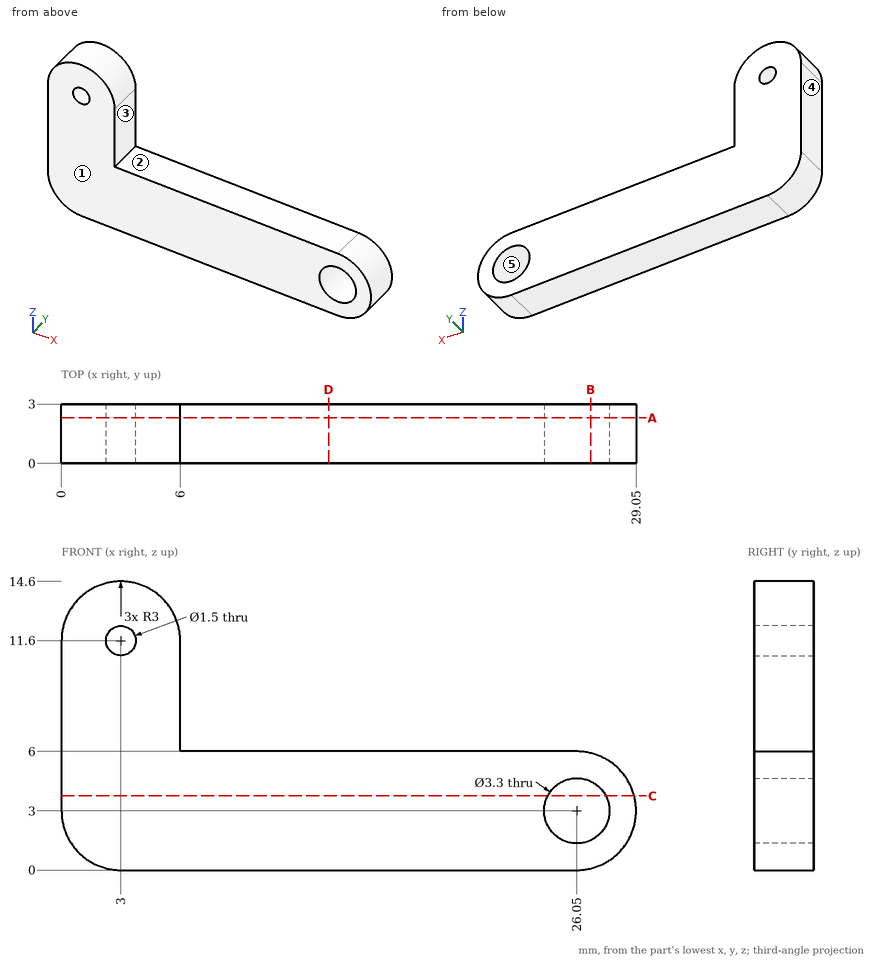
Geometry: see drawing. Coordinates: mm, zero at the bounding-box minimum. A direction names the side the tool comes from. Give positions to 0.01 mm unless a question says otherwise; leave off trailing zeros. Order: outer loops, then holes, each group sorted by start corner. A loop starts at its lowest first (then second) coordinate and runs counter-clockwise, first axis right, second up.
Q1. Ray query, probe 1 along X at (y, z) = (1.3, 3); probe 2 along X at (y, z) = (0.9, 11.6); probe 3 along X at (y, z) = (2.1, 7). Return the intervals inside material, ascending.
Checked values:
probe 1: x = 0 to 24.4, 27.7 to 29.05
probe 2: x = 0 to 2.25, 3.75 to 6
probe 3: x = 0 to 6
Q2. Section D-D on x = 13.5. Output: boundary loops of the cut face in (y, z).
Checked values:
outline: (0, 0) - (3, 0) - (3, 6) - (0, 6) - close
Q3. Section C-C on z = 3.75. Output: boundary loops of the cut face in (x, y), and give its area (3 significant figures).
Checked values:
outline: (0, 0) - (24.58, 0) - (24.58, 3) - (0, 3) - close; (27.52, 0) - (28.95, 0) - (28.95, 3) - (27.52, 3) - close
area: 78.0 mm2
Q4. Section A-A on y = 2.3. Output: boundary loops of the cut face in (x, z).
Checked values:
outline: (0, 3) arc R3 ccw to (3, 0) - (26.05, 0) arc R3 ccw to (26.05, 6) - (6, 6) - (6, 11.6) arc R3 ccw to (0, 11.6) - close; hole circle Ø1.5 at (3, 11.6); hole circle Ø3.3 at (26.05, 3)
Q5. Draft query along X for the marked faces 3, 4 and 5. Return one class per face: +X half, -X half, draft (parallel to the pull), parting line (faces both ways), or undercut.
Checked values:
face 3: +X half
face 4: -X half
face 5: undercut
Q6. Section B-B on x = 26.75. Output: boundary loops of the cut face in (y, z).
Checked values:
outline: (0, 0.08) - (3, 0.08) - (3, 1.51) - (0, 1.51) - close; (0, 4.49) - (3, 4.49) - (3, 5.92) - (0, 5.92) - close
Q7. Set-up query: the marked faces 1 and 2. Return all of +Z, -Z, +X, -X, +Y, -Y with unobstructed straight access to the full face (end or side cutting, diameter ignored); none if empty.
Checked values:
face 1: +Z, -Z, +X, -X, -Y
face 2: +Z, +X, +Y, -Y
Q8. Contact query for flat-ended pins moving along their axis: pin 1 Ø1.5 at (x, y) = (10, 0.5) entering from +Z; pin 2 Ø0.9 at (y, z) = (1, 10) entering from +X. Output: stop coordinate, or through.
Checked values:
pin 1: stops at z = 6
pin 2: stops at x = 6
